from build123d import *

# Parameters (mm, degrees)
SKETCH1_W           = 60
SKETCH1_H           = 20
BOSS_EXTRUDE1_DEPTH = 15
CUT_EXTRUDE1_DEPTH  = 22
CUT_EXTRUDE2_DEPTH  = 34


with BuildPart() as part:
    # Sketch1 → Boss-Extrude1 (new body, symmetric)
    with BuildSketch(Plane.XY):
        Rectangle(SKETCH1_W, SKETCH1_H)
    extrude(amount=BOSS_EXTRUDE1_DEPTH, both=True)

    # Sketch2 → Cut-Extrude1 (cut, symmetric)
    with BuildSketch(Plane.XY):
        Polygon((-15, -10), (-30, 10), (-30, -10), align=None)
        Polygon((15, -10), (30, 10), (30, -10), align=None)
    extrude(amount=CUT_EXTRUDE1_DEPTH, both=True, mode=Mode.SUBTRACT)

    # Sketch3 → Cut-Extrude2 (cut, symmetric)
    with BuildSketch(Plane(origin=(0, 0, 0), x_dir=(0, 0, -1), z_dir=(1, 0, 0))):
        Polygon((-15, 10), (-15, -10), (0, 10), align=None)
        Polygon((15, 10), (0, 10), (15, -10), align=None)
    extrude(amount=CUT_EXTRUDE2_DEPTH, both=True, mode=Mode.SUBTRACT)


solid = part.part
The model under review builds one solid part; all positions refer to its coordinate system, in mm. Round coordinates to 2 decimals unless told otherwise and drop trailing zeros. Write each loop counter-clockwise with the first axis right and the second up, starting at its lowest first coordinate (ties: lowest second). Pieces come first, ordered by that corner, then holes. Notation, with made-up numbers: (33.5, 66) - (38.5, 66) arc R19 cw to (38.5, 99) - close; hole circle Ø9 at (-36, -18.75). An arc over 180 degrees is marked (long way). One line per item, written item: value. Start each with the question number.
1. Consider section D-D on x = 19.5. Write out the cut boundary in (y, z).
2. Consider section B-B on y = -8. Write out the cut boundary in (x, z), and give its area (3 significant figures).
3. Consider section C-C on z = 8.25. Write out the cut boundary in (x, y).
4. Clearance check with flat-ended pins moving along their axes: P1, Ø6, axis at y = -5, z = -4.5, coming from the -X side; P2, Ø5, axis at y = 0, z = 1, coming from the -X side (3 decimals); P3, Ø6, axis at x = 6, y = -2, coming from the -Z side. State where each tip first meets the part, or that it passes through.
5. Consider section A-A on x = -11. Write out the cut boundary in (y, z), and give its area (3 significant figures).
6. The part is to be moulded in two halves that separate along X. For faces 1 (the face through (0, 2, -6)), 2 (the face through (-21, -2, 0)), 3 (the face through (21, -2, 0)), say which applies: released by +X, released by -X, zero draft, split by the parting line, or undercut.
7. To check wall thickness, follow L1, parallel to Y at x = -10, z = 4.5; L2, parallel to Y at x = 18, z = -7.75; L3, parallel to Z at x = -16.5, y = -3. State the ranges of each line that lie inside material, in increasing order. Write a range as from..to.
Checks:
1. outline: (-4, -10.5) - (10, 0) - (-4, 10.5) - close
2. outline: (-16.5, -13.5) - (16.5, -13.5) - (16.5, 13.5) - (-16.5, 13.5) - close
2. area: 891 mm^2
3. outline: (-21.75, -1) - (-15, -10) - (15, -10) - (21.75, -1) - close
4. P1: stops at x = -21
4. P2: stops at x = -24.375
4. P3: stops at z = -11.25
5. outline: (-10, -15) - (10, 0) - (-10, 15) - close
5. area: 300 mm^2
6. face 1: zero draft
6. face 2: released by -X
6. face 3: released by +X
7. L1: y = -10..4
7. L2: y = -6..-0.33
7. L3: z = -9.75..9.75
